Model file for the job. Use its own axes, mm. Face numbers are marked on the shaded views. A direction names the side the tool comes from. Coordinates: 2 decimals unless noted, no trailing zeros. Write each loop counter-clockwise with the first axis right and the second up, starting at its lowest first coordinate (ties: lowest second). Pieces come first, ordered by that corner, then holes. Notation, with made-up numbers: (47.5, -15.75) -> (70.5, -15.75) arc R16 ccw to (70.5, -11.75) -> close; hole circle Ø1 at (2, 47). An arc over 180 degrees is marked (long way). Answer as a JSON object with one key per item and string values. Group by question number.
from build123d import *

# Parameters (mm, degrees)
ESQUISSE1_R             = 15
ESQUISSE1_R_2           = 6.1
BOSS_EXTRU_1_DEPTH      = 4
ESQUISSE2_R             = 10.5
ENL_V_MAT_EXTRU_1_DEPTH = 2
CHANFREIN1_SIZE         = 0.5


with BuildPart() as part:
    # Esquisse1 → Boss.-Extru.1 (new body)
    with BuildSketch(Plane.XY):
        Circle(ESQUISSE1_R)
        Circle(ESQUISSE1_R_2, mode=Mode.SUBTRACT)
    extrude(amount=BOSS_EXTRU_1_DEPTH)

    # Esquisse2 → Enlèv. mat.-Extru.1 (cut)
    with BuildSketch(Plane.XY.offset(4)):
        Circle(ESQUISSE2_R)
    extrude(amount=-ENL_V_MAT_EXTRU_1_DEPTH, mode=Mode.SUBTRACT)

    # Chanfrein1
    chanfrein1_edges = [part.edges().sort_by_distance(p)[0] for p in [
        (-15, 0, 0),
        (-15, 0, 4),
    ]]
    chamfer(chanfrein1_edges, length=CHANFREIN1_SIZE)


solid = part.part
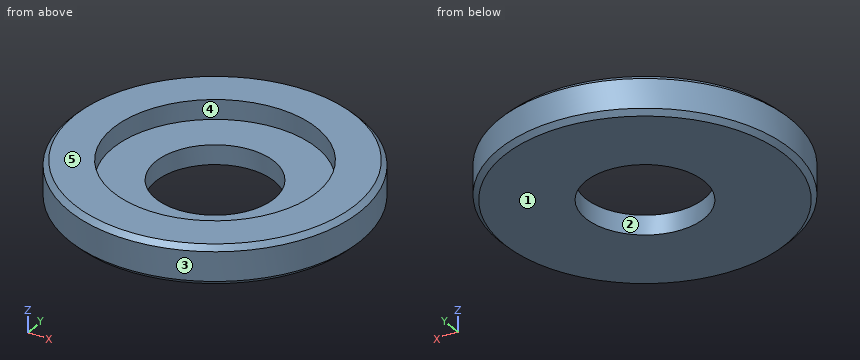
(1) 3-axis set-ups, long thin cutter, end or side, ignore diameter. For the marked faces 4 and 5: which of +Z, -Z, +X, -X, +Y, -Y reach the whole face in a straight line?
(2) Cut at D-D on z = 3.15. List the corners of the cut face in (x, y), plus the area to 3 significant figures.
(3) Cut at C-C on z = 1.15. List the corners of the cut face in (x, y), plus the area to 3 significant figures.
(4) Cut at A-A on y = 0. List the corners of the cut face in (x, z).
(5) Pin check, flat tips, straight feed: pin 1 (5 mm diameter, centred on x = -8, y = 3, fed in from +Z); pin 2 (11 mm diameter, centred on x = 0, y = 0, fed in from +Z); pin 3 (1 mm diameter, centred on x = 1, z = 1.5, fed in from -Y). Stop position of each tip, or through.
(6) Wall check: probe 1 along Y at (x, z) = (0, 0.5); probe 2 along Y at (x, z) = (0, 3.2); probe 3 along X at (y, z) = (1.5, 1.85). Give the ranges that are in metal, low to high.
(7) Pull direction X, two halves, no side cores. Call the marked faces 1, 2 and 3: released by +X, released by -X, zero draft, split by the parting line, or undercut.
Results found:
{
 "1": {"face 4": "+Z", "face 5": "+Z, +X, -X, +Y, -Y"},
 "2": {"outline": "circle Ø30 at (0, 0); hole circle Ø21 at (0, 0)", "area": "360 mm²"},
 "3": {"outline": "circle Ø30 at (0, 0); hole circle Ø12.2 at (0, 0)", "area": "590 mm²"},
 "4": {"outline": "(-15, 0.5) -> (-14.5, 0) -> (-6.1, 0) -> (-6.1, 2) -> (-10.5, 2) -> (-10.5, 4) -> (-14.5, 4) -> (-15, 3.5) -> close; (6.1, 0) -> (14.5, 0) -> (15, 0.5) -> (15, 3.5) -> (14.5, 4) -> (10.5, 4) -> (10.5, 2) -> (6.1, 2) -> close"},
 "5": {"pin 1": "stops at z = 4", "pin 2": "passes through", "pin 3": "stops at y = -14.99"},
 "6": {"probe 1": "y = -15 to -6.1, 6.1 to 15", "probe 2": "y = -15 to -10.5, 10.5 to 15", "probe 3": "x = -14.92 to -5.91, 5.91 to 14.92"},
 "7": {"face 1": "zero draft", "face 2": "undercut", "face 3": "split by the parting line"}
}
